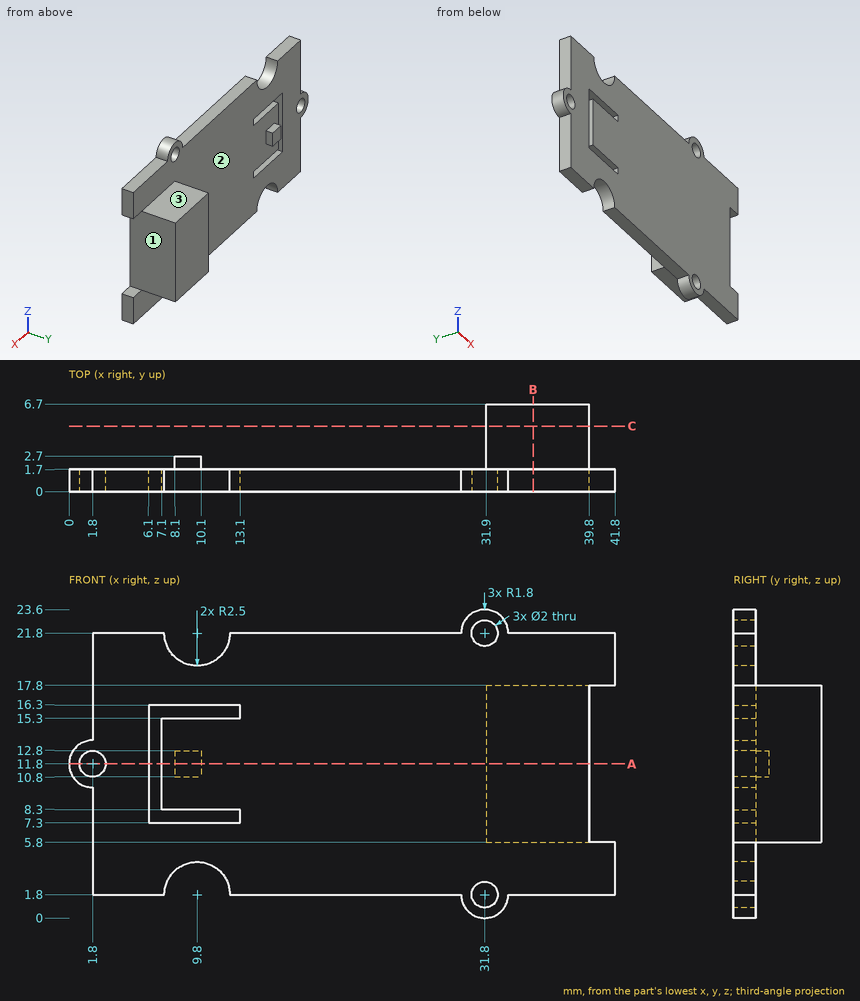
Design review of the part shown in the three views and the two pictorial views. Dimensions are in mm from the part's minimum x, y and z. Coordinates: 2 decimals unless noted, no trailing zeros. Order: outer loops, then holes, each group sorted by start corner. A loop starts at its lowest first (then second) coordinate and runs counter-clockwise, first axis right, second up. Notation, with made-up numbers: (78, -26.75) -> (94, -26.75) arc R16 ccw to (94, 3.25) -> close; hole circle Ø6 at (11.5, 6.5). An arc over 180 degrees is marked (long way). Use one line per item in the form item = value. Start each with the question number.
(1) Add section A-A on z = 11.8. State the section outline as (x, y) points, plus the area to 3 significant figures.
(2) For probe 1 along Z at (x, y) = (31.8, 0.9); probe 2 along X at (y, z) = (0.4, 11.8); probe 3 along X at (y, z) = (0.5, 11.25), list the stretches that pass through material, from the lowest coordinate up.
(3) Add section C-C on y = 5. State the section outline as (x, z) points, plus the area to 3 significant figures.
(4) Add section B-B on x = 35.5. State the section outline as (y, z) points, plus the area to 3 significant figures.
(5) Insertion check: pin 1 (1.4 mm diameter, centred on y = 1, z = 11, fed in from -X); pin 2 (0.8 mm diameter, centred on x = 41, y = 1, fed in from +Z); pin 3 (1.9 mm diameter, centred on x = 11, y = 0.5, fed in from +Z). Each pin has a flat end and moves straight along its axis. Give the tip position at first contact, or say it passes through.
(6) The part is to be moulded in two halves that separate along Z. For the marked faces 1, 2 and 3, say which applies: +Z half, -Z half, draft (parallel to the pull), parting line (faces both ways), or undercut.
Answer block:
q1.outline = (0, 0) -> (0.8, 0) -> (0.8, 1.7) -> (0, 1.7) -> close; (2.8, 0) -> (6.1, 0) -> (6.1, 1.7) -> (2.8, 1.7) -> close; (7.1, 0) -> (39.8, 0) -> (39.8, 6.7) -> (31.9, 6.7) -> (31.9, 1.7) -> (10.1, 1.7) -> (10.1, 2.7) -> (8.1, 2.7) -> (8.1, 1.7) -> (7.1, 1.7) -> close
q1.area = 104 mm²
q2.probe_1 = 0 to 0.8, 2.8 to 20.8, 22.8 to 23.6
q2.probe_2 = 0 to 0.8, 2.8 to 6.1, 7.1 to 39.8
q2.probe_3 = 0.09 to 0.96, 2.64 to 6.1, 7.1 to 39.8
q3.outline = (31.9, 5.8) -> (39.8, 5.8) -> (39.8, 17.8) -> (31.9, 17.8) -> close
q3.area = 94.8 mm²
q4.outline = (0, 1.8) -> (1.7, 1.8) -> (1.7, 5.8) -> (6.7, 5.8) -> (6.7, 17.8) -> (1.7, 17.8) -> (1.7, 21.8) -> (0, 21.8) -> close
q4.area = 94.0 mm²
q5.pin_1 = 0
q5.pin_2 = 21.8
q5.pin_3 = 20.52
q6.face_1 = undercut
q6.face_2 = draft
q6.face_3 = +Z half
